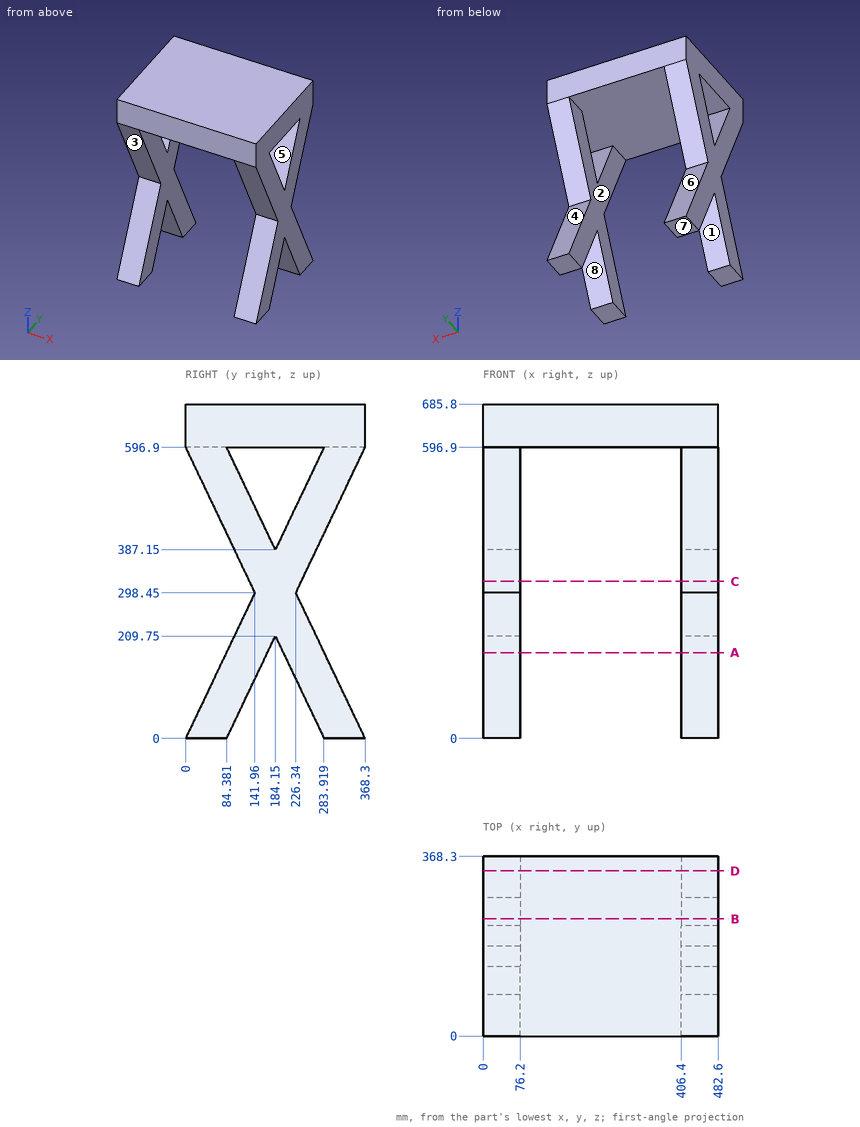
Here's the drawing with two shaded views (mm, measured from the low corner). I have some questions. A direction names the side the tool comes from. Coordinates: 2 decimals unless noted, no trailing zeros. Order: outer loops, then holes, each group sorted by start corner. A loop starts at its lowest first (then second) coordinate and runs counter-clockwise, first axis right, second up. Notation, with made-up numbers: M 52,4.5 L 77,4.5 A14 ccw 77,15.5 Z; hole C 88.5,3.25 d8. An arc over 180 degrees is marked long. Answer as CSV lines item,"result".
Item 1: On a 3-axis mill with a long thin cutter (end or side, diameter ignored), from which of +Z, -Z, +X, -X, +Y, -Y can I reach the whole of each face in a straight line? I mean the marked faces 1, 2, 3, 4 and 5. Say none if no direction works.
Results found:
face 1,"-Z, +X, -X"
face 2,"-Z, +Y, -Y"
face 3,"+X, -X, -Y"
face 4,"+X, -X, +Y"
face 5,"+X, -X"
Item 2: Imagine slicing it at B-B on y = 240. Write out the boundary of the cut face in (x, z).
Results found:
outline,"M 0,92.33 L 76.2,92.33 L 76.2,269.73 L 0,269.73 Z; M 0,327.17 L 76.2,327.17 L 76.2,504.57 L 0,504.57 Z; M 0,596.9 L 482.6,596.9 L 482.6,685.8 L 0,685.8 Z; M 406.4,92.33 L 482.6,92.33 L 482.6,269.73 L 406.4,269.73 Z; M 406.4,327.17 L 482.6,327.17 L 482.6,504.57 L 406.4,504.57 Z"
Item 3: If I drill on line 1 (X direction, y = 123.5, z = 493.5); line 2 (Z direction, x = 278, y = 353); line 3 (Y direction, x = 445, z = 425.5), over which ranges is the centre line in solid material (lowest first)?
Results found:
line 1,"0 to 76.2, 406.4 to 482.6"
line 2,"596.9 to 685.8"
line 3,"81.53 to 165.91, 202.39 to 286.77"
Item 4: For pin 1 (4 mm diameter, centred on x = 257, y = 70, fed in from -Z); pin 2 (10 mm diameter, centred on y = 39, z = 501, fed in from -X); pin 3 (1 mm diameter, centred on x = 410.5, z = 548.5, fed in from +Y) (1 decimal), each with a flat end and sliding along its axis, tell me the tip position at first contact or that it passes through.
Results found:
pin 1,"z = 596.9"
pin 2,"through"
pin 3,"y = 345.5"
Item 5: Imagine slicing it at A-A on z = 176. Write out the boundary of the cut face in (x, y) (1 decimal), plus the area to 3 significant figures.
Results found:
outline,"M 0,83.7 L 76.2,83.7 L 76.2,168.1 L 0,168.1 Z; M 0,200.2 L 76.2,200.2 L 76.2,284.6 L 0,284.6 Z; M 406.4,83.7 L 482.6,83.7 L 482.6,168.1 L 406.4,168.1 Z; M 406.4,200.2 L 482.6,200.2 L 482.6,284.6 L 406.4,284.6 Z"
area,"25,700 mm2"
Item 6: Imagine slicing it at D-D on y = 338.5. Write out the boundary of the cut face in (x, z).
Results found:
outline,"M 0,0 L 76.2,0 L 76.2,62.65 L 0,62.65 Z; M 0,534.25 L 76.2,534.25 L 76.2,596.9 L 406.4,596.9 L 406.4,534.25 L 482.6,534.25 L 482.6,685.8 L 0,685.8 Z; M 406.4,0 L 482.6,0 L 482.6,62.65 L 406.4,62.65 Z"
Item 7: We'd pull the mould along Y, two halves only. Please class the marked faces 6, 7 and 8: +Y half, -Y half, draft (parallel to the pull), parting line (faces both ways), or undercut.
Results found:
face 6,"+Y half"
face 7,"draft"
face 8,"undercut"
Item 8: Imagine slicing it at C-C on z = 322. Write out the boundary of the cut face in (x, y), plus the area to 3 significant figures.
Results found:
outline,"M 0,130.76 L 76.2,130.76 L 76.2,237.54 L 0,237.54 Z; M 406.4,130.76 L 482.6,130.76 L 482.6,237.54 L 406.4,237.54 Z"
area,"16,300 mm2"
